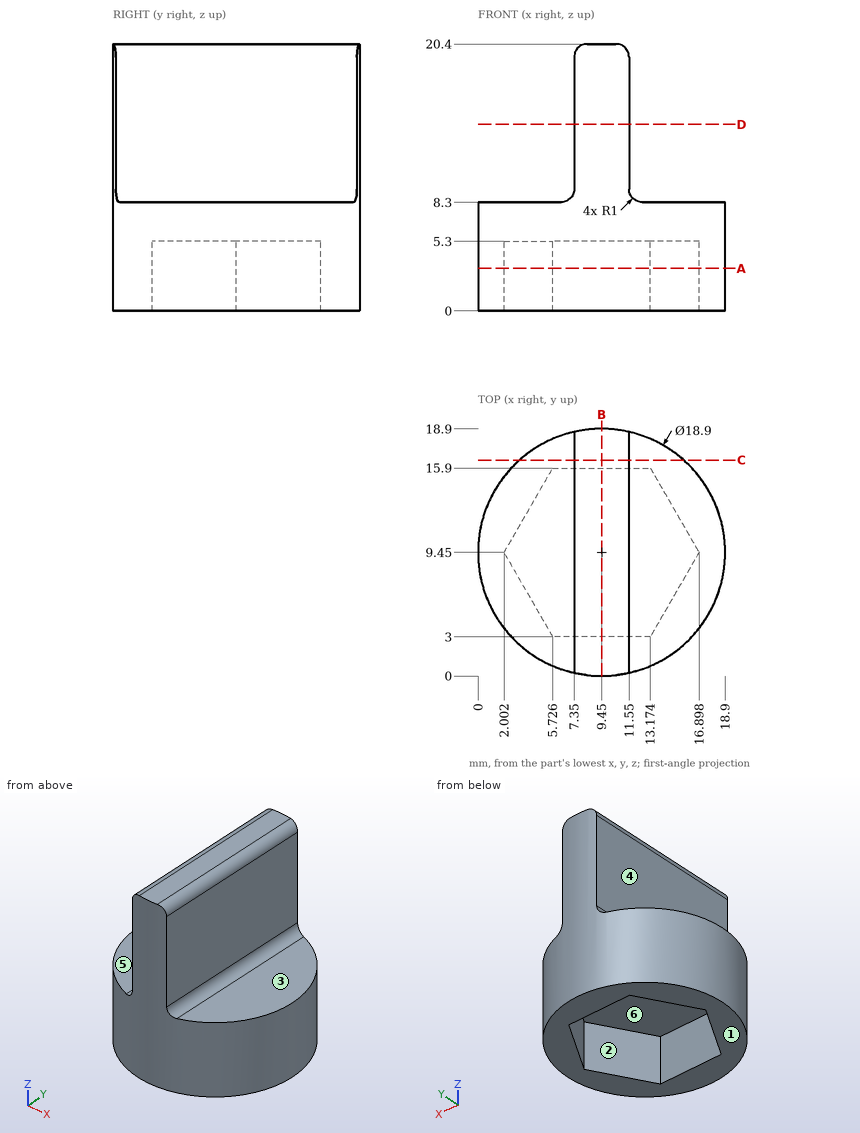
Verification items for this drawing (mm, ordinates from the low corner). A direction names the side the tool comes from. Give positions to 0.01 mm unless a question says otherwise; leave off trailing zeros. Loops run counter-clockwise (first coordinate to the right, second up) from the corner with the lowest first, then second, coordinate; pieces in that order, holes last.
(1) Depth check by flat-ended pin: pin 1 Ø6 at (x, z) = (17, 12.5) entering from +Y; pin 2 Ø8 at (y, z) = (12.5, 16.5) entering from +X; pin 3 Ø1.5 at (x, z) = (14.5, 8.5) entering from +Y; pin 4 Ø7 at (x, y) = (4.5, 6) entering from +Z. Enter the tip coordinate at first touch or a pass-through.
From the geometry:
pin 1: passes through
pin 2: stops at x = 11.55
pin 3: stops at y = 17.85
pin 4: stops at z = 20.34
(2) Section check B-B on x = 9.45. Record the cut outline in (y, z), then the cut area to 3 significant figures.
From the geometry:
outline: (0, 0) - (3, 0) - (3, 5.3) - (15.9, 5.3) - (15.9, 0) - (18.9, 0) - (18.9, 20.4) - (0, 20.4) - close
area: 317 mm2
(3) Set-up check for the marked faces 1, 2 and 3: record each of +Z, -Z, +X, -X, +Y, -Y from which the full face is reachable in a straight line by a thin tool's end or side.
From the geometry:
face 1: -Z, +X, -X, +Y, -Y
face 2: -Z
face 3: +Z, +X, +Y, -Y
(4) Section check A-A on z = 3.25. Record the cut outline in (x, y).
From the geometry:
outline: circle Ø18.9 at (9.45, 9.45); hole (2, 9.45) - (5.73, 3) - (13.17, 3) - (16.9, 9.45) - (13.17, 15.9) - (5.73, 15.9) - close
(5) Thickness scan on L1, parallel to X at y = 12.5, z = 9.25; L2, parallel to Z at x = 15.5, y = 12.5; L3, parallel to Z at x = 4, y = 8.5. Record the ranges inside material, lowest first.
From the geometry:
L1: x = 7.35 to 11.55
L2: z = 0 to 8.3
L3: z = 5.3 to 8.3
(6) Section check D-D on z = 14.25. Record the cut outline in (x, y), then the cut area to 3 significant figures.
From the geometry:
outline: (7.35, 0.24) arc R9.45 ccw to (11.55, 0.24) - (11.55, 18.66) arc R9.45 ccw to (7.35, 18.66) - close
area: 78.7 mm2
(7) Release check for a two-part mould opening along X. For the marked faces 4, 5 and 6 record: released by +X, released by -X, zero draft, split by the parting line, or undercut.
From the geometry:
face 4: released by -X
face 5: zero draft
face 6: undercut
(8) Section check C-C on y = 16.5. Record the cut outline in (x, z), then the cut area to 3 significant figures.
From the geometry:
outline: (3.16, 0) - (15.74, 0) - (15.74, 8.3) - (12.55, 8.3) arc R1 cw to (11.55, 9.3) - (11.55, 19.4) arc R1 ccw to (10.55, 20.4) - (8.35, 20.4) arc R1 ccw to (7.35, 19.4) - (7.35, 9.3) arc R1 cw to (6.35, 8.3) - (3.16, 8.3) - close
area: 155 mm2
